Autodesk Inventor part; units mm, degrees
ref_plane "YZ Plane" through (0, 0, 0) normal (1, 0, 0) x (0, 1, 0)
ref_plane "XZ Plane" through (0, 0, 0) normal (0, 1, 0) x (-1, 0, 0)
ref_plane "XY Plane" through (0, 0, 0) normal (0, 0, 1) x (1, 0, 0)
sketch "Sketch1" plane through (0, 0, 0) normal (0, 0, 1) x (1, 0, 0)
  line L0 (-36.3054, 10.7035) -> (5.6946, 10.7035)
  line L1 (5.6946, 10.7035) -> (5.6946, -24.2965)
  line L2 (5.6946, -24.2965) -> (-36.3054, -24.2965)
  line L3 (-36.3054, -24.2965) -> (-36.3054, 10.7035)
  line L4 (-37.5054, 11.9035) -> (6.8946, 11.9035)
  line L5 (6.8946, 11.9035) -> (6.8946, -25.4965)
  line L6 (6.8946, -25.4965) -> (-37.5054, -25.4965)
  line L7 (-37.5054, -25.4965) -> (-37.5054, 11.9035)
  point P0 (0, 0)
  dimension "d0" = 42
  dimension "d1" = 35
  dimension "d2" = 1.2
  dimension "d3" = 1.2
  dimension "d4" = 1.2
  dimension "d5" = 1.2
extrude "Extrusion1" add sketch "Sketch1" along normal blind 18
sketch "Sketch2" plane through (0, 0, 0) normal (0, 0, -1) x (-1, 0, 0)
  line L0 (-11.8946, 11.9035) -> (42.5054, 11.9035)
  line L1 (42.5054, 11.9035) -> (42.5054, -25.4965)
  line L2 (42.5054, -25.4965) -> (-11.8946, -25.4965)
  line L3 (-11.8946, -25.4965) -> (-11.8946, 11.9035)
  line L4 (-6.8946, -25.4965) -> (-6.8946, 11.9035)
  line L5 (37.5054, -25.4965) -> (37.5054, 11.9035)
  line L6 (37.5054, 11.9035) -> (-6.8946, 11.9035)
  line L7 (-6.8946, -25.4965) -> (37.5054, -25.4965)
  point P0 (0, 0)
  dimension "d8" = 5
  dimension "d9" = 5
extrude "Extrusion2" add sketch "Sketch2" along normal blind 2
sketch "Sketch3" plane through (0, 0, 0) normal (0, 0, 1) x (1, 0, 0)
  line L0 (-42.5054, 11.9035) -> (11.8946, 11.9035)
  line L1 (-42.5054, -25.4965) -> (-42.5054, 11.9035)
  line L2 (-37.5054, 11.9035) -> (-42.5054, 11.9035)
  line L3 (-42.5054, 11.9035) -> (-42.5054, 6.9035)
  line L4 (-42.5054, 6.9035) -> (-37.5054, 6.9035)
  line L5 (-37.5054, 6.9035) -> (-37.5054, 11.9035)
  line L6 (-37.5054, 11.9035) -> (-37.5054, -25.4965)
  line L7 (-42.5054, -25.4965) -> (-37.5054, -25.4965)
  line L8 (-37.5054, -25.4965) -> (-37.5054, -20.4965)
  line L9 (-37.5054, -20.4965) -> (-42.5054, -20.4965)
  line L10 (-42.5054, -20.4965) -> (-42.5054, -25.4965)
  line L11 (6.8946, 11.9035) -> (6.8946, -25.4965)
  line L12 (11.8946, 11.9035) -> (6.8946, 11.9035)
  line L13 (6.8946, 11.9035) -> (6.8946, 6.9035)
  line L14 (6.8946, 6.9035) -> (11.8946, 6.9035)
  line L15 (11.8946, 6.9035) -> (11.8946, 11.9035)
  line L16 (11.8946, -25.4965) -> (6.8946, -25.4965)
  line L17 (6.8946, -25.4965) -> (6.8946, -20.4965)
  line L18 (6.8946, -20.4965) -> (11.8946, -20.4965)
  line L19 (11.8946, -20.4965) -> (11.8946, -25.4965)
  point P0 (0, 0)
  dimension "d12" = 5
  dimension "d13" = 5
  dimension "d14" = 5
  dimension "d15" = 5
extrude "Extrusion3" add sketch "Sketch3" along normal blind 18 contours L18 L19 L16 L11 | L0 L15 L14 L11 | L0 L5 L4 L1 | L9 L6 L7 L1
sketch "Sketch4" plane through (0, 0, 0) normal (0, 0, 1) x (1, 0, 0)
  line L0 (-37.5054, 6.9035) -> (-42.5054, 6.9035)
  line L1 (-42.5054, 6.9035) -> (-42.5054, -20.4965)
  line L2 (-42.5054, -20.4965) -> (-37.5054, -20.4965)
  line L3 (-37.5054, -20.4965) -> (-37.5054, 6.9035)
  line L4 (6.8946, -20.4965) -> (11.8946, -20.4965)
  line L5 (11.8946, -20.4965) -> (11.8946, 6.9035)
  line L6 (11.8946, 6.9035) -> (6.8946, 6.9035)
  line L7 (6.8946, 6.9035) -> (6.8946, -20.4965)
  point P0 (0, 0)
extrude "Extrusion4" cut sketch "Sketch4" against normal blind 18
chamfer "Chamfer1" distance 2 angle 45 4 edges at (-37.5054, 6.9035, 8) (-37.5054, -20.4965, 8) (6.8946, 6.9035, 8) (6.8946, -20.4965, 8)
sketch "Sketch5" plane through (0, 0, 18) normal (0, 0, 1) x (1, 0, 0)
  line L0 (5.6946, 10.7035) -> (5.6946, -24.2965)
  line L1 (8.8946, -20.4965) -> (5.6946, -20.4965)
  line L2 (5.6946, -20.4965) -> (5.6946, -5.4965)
  line L3 (5.6946, -5.4965) -> (8.8946, -5.4965)
  line L4 (8.8946, -5.4965) -> (8.8946, -20.4965)
  point P0 (0, 0)
  dimension "d23" = 15
extrude "Extrusion5" cut sketch "Sketch5" against normal blind 10
sketch "Sketch6" plane through (0, 0, 18) normal (0, 0, 1) x (1, 0, 0)
  line L0 (11.8946, 11.9035) -> (-42.5054, 11.9035)
  line L1 (-42.5054, 11.9035) -> (-42.5054, 6.9035)
  line L2 (-39.5054, -20.4965) -> (-42.5054, -20.4965)
  line L3 (-42.5054, -20.4965) -> (-42.5054, -25.4965)
  line L4 (-42.5054, -25.4965) -> (11.8946, -25.4965)
  line L5 (11.8946, -25.4965) -> (11.8946, -20.4965)
  line L6 (8.8946, 6.9035) -> (11.8946, 6.9035)
  line L7 (11.8946, 6.9035) -> (11.8946, 11.9035)
  point P0 (0, 0)
  point P1 (-40.0054, 9.4035)
  point P2 (-40.0054, -22.9965)
  point P3 (9.3946, -22.9965)
  point P4 (9.3946, 9.4035)
  dimension "d26" = 2.5
  dimension "d27" = 2.5
  dimension "d28" = 2.5
  dimension "d29" = 2.5
  dimension "d30" = 2.5
  dimension "d31" = 2.5
  dimension "d32" = 2.5
  dimension "d33" = 2.5
  dimension "d34" = 49.4
  dimension "d35" = 32.4
hole "Hole1" at (-40.0054, 9.4035, 18) at (-40.0054, -22.9965, 18) at (9.3946, -22.9965, 18) at (9.3946, 9.4035, 18) direction (0, 0, -1) diameter 2 depth 8 tip angle 118
sketch "Sketch7" plane through (-37.5054, -18.4965, 18) normal (-1, 0, 0) x (0, 0, 1)
  line L0 (-20, 0) -> (-10, 0)
  line L1 (0, 23.4) -> (-18, 23.4)
  line L2 (-18, 23.4) -> (-18, 0)
  line L3 (-18, 0) -> (0, 0)
  line L4 (0, 0) -> (0, 23.4)
  line L5 (-18, 29.2) -> (-18, -5.8)
  point P0 (-18, 18.4965)
extrude "Extrusion6" cut sketch "Sketch7" against normal blind 2
properties part number "main body"
Here's how the part is built. I have some questions about the finished solid (model axes, mm). A direction names the side the tool comes from. Round coordinates to 2 decimals unless told otherwise and drop trailing zeros. Loops run counter-clockwise (first coordinate to the right, second up) from the corner with the lowest first, then second, coordinate; pieces in that order, holes last. Notation, with made-up numbers: (49, 65) - (54, 65) arc R9 ccw to (54, 75) - close; hole circle Ø6 at (51, 31.25). An arc over 180 degrees is marked (long way). One line per question, with ' | ' between items. Start each with the question number.
Q1. For faces 1 (the flat face through (-41, -20.496, 8)), 2 (the flat face through (6, -5.496, 13)), 3 (the flat face through (6, -13, 8)), 4 (the flat face through (-16, 10.704, 9)), which set-ups out of +Z, -Z, +X, -X, +Y, -Y let a thin tool reach every point of the face, with its end or its side?
Q2. We'd pull the mould along X, two halves only. Please class faces 5 (the flat face through (6.895, -4, 6)), 6 (the flat face through (-42.505, -23, 8)), 7 (the cylindrical face through (-41, 9.5, 13.9)): +X half, -X half, draft (parallel to the pull), parting line (faces both ways), or undercut.
Q3. I want a section at C-C (z = 3.5). Write out the boundary of the cut face in (x, y), then the cut area to 3 significant figures.
Q4. I want a section at A-A (z = 12.75). Write out the boundary of the cut face in (x, y).
Q5. Will these pins go through, and if not, where does the flat tip stop? pin 1 (17.5 mm diameter, centred on x = -13, y = 1, fed in from +Z); pin 2 (1.6 mm diameter, centred on x = -40.01, y = 9.4, fed in from +Z); pin 3 (5 mm diameter, centred on y = -14.5, z = 4.5, fed in from +X).
Q6. I want a section at D-D (y = -10). Write out the boundary of the cut face in (x, z), then the cut area to 3 significant figures.
Q7. I want a section at B-B (x = -30). Write out the boundary of the cut face in (y, z), then the cut area to 3 significant figures.
Q8. Please list where these lines run through material, in increasing order: line 1 (Y direction, x = -37, z = 13); line 2 (Y direction, x = 0, z = 15.25); line 3 (X direction, y = -23, z = 6.5). Write a range as [from, to].
Response values:
1) face 1: +Z, -Z, -X | face 2: +Z, +X, -X | face 3: +Z, +X | face 4: +Z
2) face 5: +X half | face 6: -X half | face 7: undercut
3) outline: (-42.51, -25.5) - (11.89, -25.5) - (11.89, -20.5) - (8.89, -20.5) - (6.89, -18.5) - (6.89, 4.9) - (8.89, 6.9) - (11.89, 6.9) - (11.89, 11.9) - (-42.51, 11.9) - (-42.51, 6.9) - (-39.51, 6.9) - (-37.51, 4.9) - (-36.31, 4.9) - (-36.31, 10.7) - (5.69, 10.7) - (5.69, -24.3) - (-36.31, -24.3) - (-36.31, -18.5) - (-37.51, -18.5) - (-39.51, -20.5) - (-42.51, -20.5) - close | area: 270 mm²
4) outline: (-42.51, -25.5) - (11.89, -25.5) - (11.89, -20.5) - (5.69, -20.5) - (5.69, -24.3) - (-36.31, -24.3) - (-36.31, -18.5) - (-37.51, -18.5) - (-39.51, -20.5) - (-42.51, -20.5) - close; (-42.51, 6.9) - (-39.51, 6.9) - (-37.51, 4.9) - (-36.31, 4.9) - (-36.31, 10.7) - (5.69, 10.7) - (5.69, -5.5) - (6.89, -5.5) - (6.89, 4.9) - (8.89, 6.9) - (11.89, 6.9) - (11.89, 11.9) - (-42.51, 11.9) - close; hole circle Ø2 at (-40.01, -23); hole circle Ø2 at (-40.01, 9.4); hole circle Ø2 at (9.39, -23); hole circle Ø2 at (9.39, 9.4)
5) pin 1: stops at z = 0 | pin 2: stops at z = 9.88 | pin 3: stops at x = 6.89
6) outline: (-37.51, -2) - (6.89, -2) - (6.89, 8) - (5.69, 8) - (5.69, 0) - (-37.51, 0) - close | area: 98.4 mm²
7) outline: (-25.5, -2) - (11.9, -2) - (11.9, 18) - (10.7, 18) - (10.7, 0) - (-24.3, 0) - (-24.3, 18) - (-25.5, 18) - close | area: 118 mm²
8) line 1: y = [-25.5, -18.5], [4.9, 11.9] | line 2: y = [-25.5, -24.3], [10.7, 11.9] | line 3: x = [-42.51, -36.31], [5.69, 11.89]
